```python
from build123d import *

# Parameters (mm, degrees)
F2_R     = 310
F3_DEPTH = 800
F4_W     = 400
F4_H     = 250
F5_DEPTH = 323.001
F6_DEPTH = 323.001


with BuildPart() as f1:
    # F0 (on Front) → F1 (revolve)
    with BuildSketch(Plane.XZ):
        Polygon((0, 1130), (0, 0), (30, 0), (30, 75), (230, 75), (230, 0), (260, 0), (260, 75), (323, 255), (323, 1070), (318, 1070), (318, 1120), (323, 1120), (323, 1130), align=None)
    revolve(axis=Axis((0, 0, 565), (0, 0, 1)))

    # F2 (on face) → F3 (cut)
    with BuildSketch(Plane.XY.offset(1130)):
        Circle(F2_R)
    extrude(amount=-F3_DEPTH, mode=Mode.SUBTRACT)

    # F4 (on Right) → F5 (cut, through all)
    with BuildSketch(Plane.YZ):
        with Locations((0, 75)):
            Rectangle(F4_W, F4_H)
    extrude(amount=-F5_DEPTH, mode=Mode.SUBTRACT)

    # F4 (on Right) → F6 (cut, through all)
    with BuildSketch(Plane.YZ):
        with Locations((0, 75)):
            Rectangle(F4_W, F4_H)
    extrude(amount=F6_DEPTH, mode=Mode.SUBTRACT)


solid = f1.part
```
Geometry: final body of the model. Coordinates: model frame, mm. A direction names the side the tool comes from. Round coordinates to 2 decimals unless told otherwise and drop trailing zeros. Write each loop counter-clockwise with the first axis right and the second up, starting at its lowest first coordinate (ties: lowest second). Pieces come first, ordered by that corner, then holes. Notation, with made-up numbers: M 87.25,13 L 146.25,13 A5 ccw 146.25,21 Z; hole C 27,43.25 d3. An arc over 180 degrees is marked long. Answer in a Markdown table with one row per item. Add a question column.
(1) Draft query along Y for faces 6 (the face through (2, -211, 75)), 7 (the face through (-41.397, 315.294, 1095.35)), 8 (the face through (2, -236, 0)). Return one class per face: pulls with the +Y half, pulls with the -Y half, needs draft (parallel to the pull), parting line crosses it, or undercut.
(2) Cut plane C-C, the plane z = 996.5. Return the cut outline in (x, y), then the cut area to 3 significant figures.
(3) Reachability of faces 1 (the face through (238, -214, 1070)), 2 (the face through (4, -3, 200)), 3 (the face through (1.663, 229.994, 36.975)), 4 (the face through (-67.2, -302.63, 735.6)), 5 (the face through (-2.523, -259.988, 38.025)) from +Z, -Z, +X, -X, +Y, -Y: full face, straight path, thin tool, end or side. Return the list, or none.
(4) Cut plane A-A, the plane x = 0. Return the cut outline in (y, z).
(5) Ray query, L1, parallel to Y at x = 0, z = 628; L2, parallel to X at y = -166, z = 1028; L3, parallel to Z at x = 7, y = 224.5. Return the intervals inside material, ascending.
(6) Cut plane B-B, the plane y = 0. Return the cut outline in (x, z).
(7) Contact query for flat-ended pins moving along their axis: pin 1 (6 mm diameter, centred on y = 119, z = 412.5, fed in from +X); pin 2 (10 mm diameter, centred on x = -82.5, y = 15, fed in from +Z); pin 3 (2 mm diameter, centred on y = 72.5, z = 508.5, fed in from +X). Output: stop coordinate, or through.
Established:
| question | item | result |
|---|---|---|
| 1 | face 6 | undercut |
| 1 | face 7 | parting line crosses it |
| 1 | face 8 | needs draft |
| 2 | outline | C 0,0 d646; hole C 0,0 d620 |
| 2 | area | 25,900 mm² |
| 3 | face 1 | none |
| 3 | face 2 | -Z, +X, -X |
| 3 | face 3 | -Z |
| 3 | face 4 | +Z |
| 3 | face 5 | -Z, -Y |
| 4 | outline | M -323,255 L -260,75 L -260,0 L -230,0 L -230,75 L -200,75 L -200,200 L 200,200 L 200,75 L 230,75 L 230,0 L 260,0 L 260,75 L 323,255 L 323,1070 L 318,1070 L 318,1120 L 323,1120 L 323,1130 L 310,1130 L 310,330 L -310,330 L -310,1130 L -323,1130 L -323,1120 L -318,1120 L -318,1070 L -323,1070 Z |
| 5 | L1 | -323 to -310, 310 to 323 |
| 5 | L2 | -277.08 to -261.81, 261.81 to 277.08 |
| 5 | L3 | 75 to 330 |
| 6 | outline | M -323,255 L -303.75,200 L 303.75,200 L 323,255 L 323,1070 L 318,1070 L 318,1120 L 323,1120 L 323,1130 L 310,1130 L 310,330 L -310,330 L -310,1130 L -323,1130 L -323,1120 L -318,1120 L -318,1070 L -323,1070 Z |
| 7 | pin 1 | x = 301.45 |
| 7 | pin 2 | z = 330 |
| 7 | pin 3 | x = 314.99 |
